Design review of the part built by this model. Coordinates are the model's own, in mm. Face numbers are marked on the shaded views. A direction names the side the tool comes from. Round coordinates to 2 decimals unless told otherwise and drop trailing zeros. Loops run counter-clockwise (first coordinate to the right, second up) from the corner with the lowest first, then second, coordinate; pieces in that order, holes last. Notation, with made-up numbers: M -28.5,-4 L 17.5,-4 A14 cw 17.5,8 Z; hole C 55.5,29.5 d10. An arc over 180 degrees is marked long. One line per item, written item: value. Start each with the question number.
Item 1: Mouldability with a two-part tool opening along X and no side actions: class the marked faces 3, 4 and 5 as released by +X, released by -X, zero draft, split by the parting line, or undercut.
Item 2: Clearance check with flat-ended pins moving along their axes: pin 1 (13.5 mm diameter, centred on x = -77.5, z = 29, fed in from -Y); pin 2 (2 mm diameter, centred on x = -34.5, y = 24.5, fed in from +Z); pin 3 (12 mm diameter, centred on y = 15.5, z = 10, fed in from -X). State where each tip first meets the part, or that it passes through.
Item 3: We need section C-C (y = 33). Write out the cut boundary in (x, z), then the cut area to 3 significant figures.
Item 4: We need section A-A (y = -31.5). Write out the cut boundary in (x, z).
Item 5: For line 1 along X through (y, z) = (33.5, 29); line 2 along X through (y, z) = (-4, 27); line 3 along X through (y, z) = (27.5, 21.5), list the stretches that pass through material, from the lowest coordinate up.
Item 6: For the marked faces 1 and 2, list the 3-axis set-ups (+Z, -Z, +X, -X, +Y, -Y) from which the entire face can be reached by the end or side of a thin tool; tool diameter is ignored.
Item 7: We need section B-B (z = 29). State how many separate pieces and enclosed holes the cut face has, then the cut area to 3 significant figures.
Item 8: We need section D-D (x = -32). Write out the cut boundary in (y, z), then the cut area to 3 significant figures.
from build123d import *

# Parameters (mm, degrees)
SKETCH1_W                      = 190
SKETCH1_H                      = 90
BOSS_EXTRUDE1_DEPTH            = 5
SKETCH2_W                      = 3.9
SKETCH2_H                      = 90
BOSS_EXTRUDE2_DEPTH            = 30
SKETCH3_W                      = 34
SKETCH3_H                      = 5
SKETCH3_W_2                    = 47
BOSS_EXTRUDE3_DEPTH            = 90
SKETCH4_W                      = 182.2
SKETCH4_H                      = 6
CUT_EXTRUDE1_DEPTH             = 5
CHAMFER6_SIZE                  = 20
BOSS_EXTRUDE4_DEPTH            = 78
FILLET5_R                      = 2
SKETCH9_R                      = 6.5
CUT_EXTRUDE4_DEPTH             = 10
SKETCH10_R                     = 7.55
CUT_EXTRUDE5_DEPTH             = 4
SKETCH15_R                     = 2.35
CUT_EXTRUDE7_DEPTH             = 8
CHAMFER7_SIZE                  = 1
SKETCH17_R                     = 6.1
CUT_EXTRUDE8_DEPTH             = 3.2
FILLET7_R                      = 0.2
CHAMFER8_SIZE                  = 9.9
CUT_EXTRUDE9_REACH             = 164.433
SKETCH18_W                     = 5
SKETCH18_H                     = 78
CUT_EXTRUDE9_DIRECTION_2_REACH = 164.433
BOSS_EXTRUDE5_DEPTH            = 78
FILLET8_R                      = 5


with BuildPart() as part:
    # Sketch1 → Boss-Extrude1 (new body)
    with BuildSketch(Plane.XY):
        Rectangle(SKETCH1_W, SKETCH1_H)
    extrude(amount=BOSS_EXTRUDE1_DEPTH)

    # Sketch2 → Boss-Extrude2 (add)
    with BuildSketch(Plane.XY.offset(5)):
        with Locations((-93.05, 0)):
            Rectangle(SKETCH2_W, SKETCH2_H)
        with Locations((93.05, 0)):
            Rectangle(SKETCH2_W, SKETCH2_H)
    extrude(amount=BOSS_EXTRUDE2_DEPTH)

    # Sketch3 → Boss-Extrude3 (add)
    with BuildSketch(Plane(origin=(0, 45, 0), x_dir=(1, 0, 0), z_dir=(0, 1, 0))):
        with Locations((-74.1, -16.5)):
            Rectangle(SKETCH3_W, SKETCH3_H)
        with Locations((67.6, -16.5)):
            Rectangle(SKETCH3_W_2, SKETCH3_H)
    extrude(amount=-BOSS_EXTRUDE3_DEPTH)

    # Sketch4 → Cut-Extrude1 (cut)
    with BuildSketch(Plane.XY.offset(19)):
        with Locations((0, 42)):
            Rectangle(SKETCH4_W, SKETCH4_H)
        with Locations((0, -42)):
            Rectangle(SKETCH4_W, SKETCH4_H)
    extrude(amount=-CUT_EXTRUDE1_DEPTH, mode=Mode.SUBTRACT)

    # Chamfer6
    # the kernel refuses this chamfer: 20 mm, written as the material it adds along each edge
    with BuildSketch(Plane(origin=(-91.1, 45, 5), x_dir=(0.9996219169112968, 0, -0.02749587661058636), z_dir=(0, -1, 0))) as chamfer6_piece_1:
        Polygon((CHAMFER6_SIZE * 0.999621916911, CHAMFER6_SIZE * 0.0274958766106), (-CHAMFER6_SIZE * 0.0274958766106, CHAMFER6_SIZE * 0.999621916911), (0, 0), align=None)
    extrude(amount=90)
    with BuildSketch(Plane(origin=(91.1, -45, 5), x_dir=(0.027495876610586317, 0, 0.9996219169112968), z_dir=(0, 1, 0))) as chamfer6_piece_2:
        Polygon((CHAMFER6_SIZE * 0.999621916911, -CHAMFER6_SIZE * 0.0274958766106), (-CHAMFER6_SIZE * 0.0274958766106, -CHAMFER6_SIZE * 0.999621916911), (0, 0), align=None)
    extrude(amount=90)
    # the kernel refuses this chamfer: 20 mm, written as the material it takes off along each edge
    with BuildSketch(Plane(origin=(-95, -96.433659759, 0), x_dir=(0.9996219169112968, 0, -0.027495876610586372), z_dir=(0, 1, 0)), Plane(origin=(95, 96.433659759, 0), x_dir=(-0.9996219169112968, 0, -0.027495876610586372), z_dir=(0, -1, 0))) as chamfer6_2_piece_1:
        Polygon((CHAMFER6_SIZE * 0.999621916911, -CHAMFER6_SIZE * 0.0274958766106), (-CHAMFER6_SIZE * 0.0274958766106, -CHAMFER6_SIZE * 0.999621916911), (0, 0), align=None)
    extrude(amount=192.867319519, mode=Mode.SUBTRACT)

    # Sketch7 → Boss-Extrude4 (add)
    with BuildSketch(Plane(origin=(0, 39, 0), x_dir=(1, 0, 0), z_dir=(0, 1, 0))):
        Polygon((-85.1, -19), (-91.1, -25), (-91.1, -35), (-68.1, -35), (-68.1, -19), align=None)
        Polygon((68.1, -35), (68.1, -19), (85.1, -19), (91.1, -25), (91.1, -35), align=None)
    extrude(amount=-BOSS_EXTRUDE4_DEPTH)

    # Fillet5
    fillet5_edges = [part.edges().sort_by_distance(p)[0] for p in [
        (-68.1, 0, 35),
        (68.1, 0, 35),
    ]]
    fillet(fillet5_edges, radius=FILLET5_R)

    # Sketch9 → Cut-Extrude4 (cut)
    with BuildSketch(Plane.XY.offset(35)):
        with Locations((-82.45, -0.90743758)):
            Circle(SKETCH9_R)
        with Locations(Location((82.45, -0.90743758, 0), (0, 0, 180))):
            Circle(SKETCH9_R)
    extrude(amount=-CUT_EXTRUDE4_DEPTH, mode=Mode.SUBTRACT)

    # Sketch10 → Cut-Extrude5 (cut)
    with BuildSketch(Plane.XY.offset(35)):
        with Locations((-82.45, -0.90743758)):
            Circle(SKETCH10_R)
        with Locations((82.45, -0.90743758)):
            Circle(SKETCH10_R)
    extrude(amount=-CUT_EXTRUDE5_DEPTH, mode=Mode.SUBTRACT)

    # Sketch15 → Cut-Extrude7 (cut)
    with BuildSketch(Plane(origin=(0, 39, 0), x_dir=(1, 0, 0), z_dir=(0, 1, 0))):
        with Locations(Location((75.766666667, -21, 0), (0, 0, 270))):
            Circle(SKETCH15_R)
        with Locations(Location((-75.766666667, -21, 0), (0, 0, 90))):
            Circle(SKETCH15_R)
        with Locations(Location((78.766666667, -29, 0), (0, 0, 270))):
            Circle(SKETCH15_R)
        with Locations(Location((-78.766666667, -29, 0), (0, 0, 90))):
            Circle(SKETCH15_R)
    extrude(amount=-CUT_EXTRUDE7_DEPTH, mode=Mode.SUBTRACT)

    # Chamfer7
    chamfer7_edges = [part.edges().sort_by_distance(p)[0] for p in [
        (-75.766666667, 39, 23.35),
        (78.766666667, 39, 26.65),
        (-78.766666667, 39, 31.35),
        (75.766666667, 39, 18.65),
    ]]
    chamfer(chamfer7_edges, length=CHAMFER7_SIZE)

    # Sketch17 → Cut-Extrude8 (cut)
    with BuildSketch(Plane.XZ.offset(39)):
        with Locations((79.6, 27)):
            Circle(SKETCH17_R)
        with Locations(Location((-79.6, 27, 0), (0, 0, 180))):
            Circle(SKETCH17_R)
    extrude(amount=-CUT_EXTRUDE8_DEPTH, mode=Mode.SUBTRACT)

    # Fillet7
    fillet7_edges = [part.edges().sort_by_distance(p)[0] for p in [
        (73.5, -39, 27),
        (-73.5, -39, 27),
    ]]
    fillet(fillet7_edges, radius=FILLET7_R)

    # Chamfer8
    # the kernel refuses this chamfer: 9.9 mm, written as the material it takes off along each edge
    with BuildSketch(Plane(origin=(-95, 45, -5.459661581), x_dir=(0.9996219169112968, 0.027495876610586265, 0), z_dir=(0, 0, 1)), Plane(origin=(95, 45, 60.459661581), x_dir=(-0.9996219169112968, 0.02749587661058615, 0), z_dir=(0, 0, -1))) as chamfer8_piece_1:
        Polygon((CHAMFER8_SIZE * 0.999621916911, -CHAMFER8_SIZE * 0.0274958766106), (-CHAMFER8_SIZE * 0.0274958766106, -CHAMFER8_SIZE * 0.999621916911), (0, 0), align=None)
    extrude(amount=65.919323162, mode=Mode.SUBTRACT)

    # Cut-Extrude9: up to this face of the body (flat: up to its plane)
    cut_extrude9_end = Plane(part.part.faces().sort_by_distance((-68.1, 0, 26))[0])
    # Sketch18 → Cut-Extrude9 (cut, up to the picked face)
    with BuildSketch(Plane(origin=(-57.1, 0, 0), x_dir=(0, 0, -1), z_dir=(1, 0, 0)), mode=Mode.PRIVATE) as cut_extrude9_sk1:
        with Locations((-16.5, 0)):
            Rectangle(SKETCH18_W, SKETCH18_H)
    cut_extrude9_tool1 = split(extrude(cut_extrude9_sk1.sketch, amount=-CUT_EXTRUDE9_REACH, mode=Mode.PRIVATE), bisect_by=cut_extrude9_end, keep=Keep.BOTH, mode=Mode.PRIVATE)
    add(cut_extrude9_tool1.solids().sort_by(Axis((-57.1, 0, 16.5), (-1, 0, 0)))[0], mode=Mode.SUBTRACT)

    # Cut-Extrude9 direction 2: up to this face of the body (flat: up to its plane)
    cut_extrude9_direction_2_end = Plane(part.part.faces().sort_by_distance((68.1, 0, 26))[0])
    # Sketch18 → Cut-Extrude9 direction 2 (cut, up to the picked face)
    with BuildSketch(Plane(origin=(-57.1, 0, 0), x_dir=(0, 0, -1), z_dir=(1, 0, 0)), mode=Mode.PRIVATE) as cut_extrude9_direction_2_sk1:
        with Locations((-16.5, 0)):
            Rectangle(SKETCH18_W, SKETCH18_H)
    cut_extrude9_direction_2_tool1 = split(extrude(cut_extrude9_direction_2_sk1.sketch, amount=CUT_EXTRUDE9_DIRECTION_2_REACH, mode=Mode.PRIVATE), bisect_by=cut_extrude9_direction_2_end, keep=Keep.BOTH, mode=Mode.PRIVATE)
    add(cut_extrude9_direction_2_tool1.solids().sort_by(Axis((-57.1, 0, 16.5), (1, 0, 0)))[0], mode=Mode.SUBTRACT)

    # Sketch20 → Boss-Extrude5 (add)
    with BuildSketch(Plane(origin=(0, 39, 0), x_dir=(1, 0, 0), z_dir=(0, 1, 0))):
        Polygon((-68.1, -14), (-68.1, -5), (-71.1, -5), (-80.1, -14), align=None)
        Polygon((71.1, -5), (80.1, -14), (68.1, -14), (68.1, -5), align=None)
    extrude(amount=-BOSS_EXTRUDE5_DEPTH)

    # Fillet8
    fillet8_edges = [part.edges().sort_by_distance(p)[0] for p in [
        (-68.1, 0, 5),
        (68.1, 0, 5),
    ]]
    fillet(fillet8_edges, radius=FILLET8_R)


solid = part.part
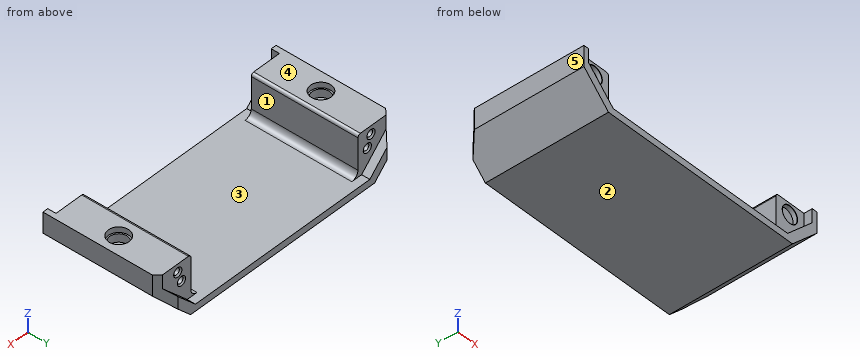
A:
1. face 3: undercut
1. face 4: zero draft
1. face 5: released by -X
2. pin 1: y = -39
2. pin 2: z = 5
2. pin 3: x = -91
3. outline: M -95,20 L -75,0 L 75,0 L 95,20 L 95,35 L 70.1,35 A2 ccw 68.1,33 L 68.1,10 A5 cw 63.1,5 L -63.1,5 A5 cw -68.1,10 L -68.1,33 A2 ccw -70.1,35 L -95,35 Z; hole C -78.77,29 d4.7; hole C -75.77,21 d4.7; hole C 75.77,21 d4.7; hole C 78.77,29 d4.7
3. area: 2,100 mm2
4. outline: M -95,20 L -75,0 L 75,0 L 95,20 L 95,35 L 70.1,35 A2 ccw 68.1,33 L 68.1,10 A5 cw 63.1,5 L -63.1,5 A5 cw -68.1,10 L -68.1,33 A2 ccw -70.1,35 L -95,35 Z
5. line 1: -95 to -81.12, -76.42 to -68.1, 68.1 to 76.42, 81.12 to 95
5. line 2: -95 to -88.17, -76.73 to -68.1, 68.1 to 76.73, 88.17 to 95
5. line 3: -95 to -68.1, 68.1 to 95
6. face 1: +Z, +Y, -Y
6. face 2: -Z, +X, -X, +Y, -Y
7. separate pieces: 2
7. enclosed holes: 2
7. area: 3,810 mm2
8. outline: M -45,0 L 45,0 L 45,5 L -45,5 Z
8. area: 450 mm2
